```python
from build123d import *

# Parameters (mm, degrees)
F0_R           = 30
F1_DEPTH       = 6
F2_R           = 27
F3_DEPTH       = 0.55
F4_R           = 0.75
F5_DEPTH       = 30.001
F5_DEPTH_BACK  = 30.001
F6_R           = 20
F7_DEPTH       = 5.4510001
F8_R           = 0.75
F9_DEPTH       = 30.0010001
F9_DEPTH_BACK  = 30.0010001
F11_DEPTH      = 3.95
F11_DEPTH_BACK = 0.5510001
F13_DEPTH      = 4.5
F14_R          = 2.05
F15_DEPTH      = 1.5010001


with BuildPart() as f1:
    # F0 (on Top) → F1 (new body)
    with BuildSketch(Plane.XY):
        Circle(F0_R)
    extrude(amount=F1_DEPTH)

    # F2 (on face) → F3 (cut)
    with BuildSketch(Plane.XY.offset(6)):
        Circle(F2_R)
    extrude(amount=-F3_DEPTH, mode=Mode.SUBTRACT)

    # F4 (on Front) → F5 (cut, two sides)
    with BuildSketch(Plane.XZ) as f5_sk:
        with Locations((0, 2.2661738681)):
            Circle(F4_R)
    extrude(amount=-F5_DEPTH, mode=Mode.SUBTRACT)
    extrude(f5_sk.sketch, amount=F5_DEPTH_BACK, mode=Mode.SUBTRACT)

    # F6 (on face) → F7 (cut, through all)
    with BuildSketch(Plane.XY.offset(5.45)):
        Circle(F6_R)
    extrude(amount=-F7_DEPTH, mode=Mode.SUBTRACT)

    # F8 (on Right) → F9 (cut, two sides)
    with BuildSketch(Plane.YZ) as f9_sk:
        with Locations((0, 4)):
            Circle(F8_R)
    extrude(amount=-F9_DEPTH, mode=Mode.SUBTRACT)
    extrude(f9_sk.sketch, amount=F9_DEPTH_BACK, mode=Mode.SUBTRACT)

    # F10 (on face) → F11 (cut, two sides)
    with BuildSketch(Plane.XY.offset(5.45)) as f11_sk:
        with BuildLine():
            ThreePointArc((-24.9057688902, 10.4260575477), (-28.0026498746, 7.54), (-26.7736042577, 3.4891424523))
            ThreePointArc((-26.7736042577, 3.4891424523), (-26.0714326419, 7.02), (-24.9057688902, 10.4260575477))
        make_face()
        with BuildLine():
            ThreePointArc((24.9057688902, -10.4260575477), (26.0714326419, -7.02), (26.7736042577, -3.4891424523))
            ThreePointArc((26.7736042577, -3.4891424523), (20.2777809437, -5.46), (24.9057688902, -10.4260575477))
        make_face()
    extrude(amount=-F11_DEPTH, mode=Mode.SUBTRACT)
    extrude(f11_sk.sketch, amount=F11_DEPTH_BACK, mode=Mode.SUBTRACT)

    # F12 (on face) → F13 (cut)
    with BuildSketch(Plane.XY.offset(6)):
        with BuildLine():
            ThreePointArc((-26.7736042577, 3.4891424523), (-22.4869694193, 2.8576411905), (-20.1402154091, 6.5))
            ThreePointArc((-20.1402154091, 6.5), (-21.5968135459, 9.587249093), (-24.9057688902, 10.4260575477))
            ThreePointArc((-24.9057688902, 10.4260575477), (-28.0026498746, 7.54), (-26.7736042577, 3.4891424523))
        make_face()
        with BuildLine():
            ThreePointArc((26.7736042577, -3.4891424523), (26.0714326419, -7.02), (24.9057688902, -10.4260575477))
            ThreePointArc((24.9057688902, -10.4260575477), (27.2274645021, -9.0434018632), (28.1402154091, -6.5))
            ThreePointArc((28.1402154091, -6.5), (27.7825742186, -4.8467540102), (26.7736042577, -3.4891424523))
        make_face()
    extrude(amount=-F13_DEPTH, mode=Mode.SUBTRACT)

    # F14 (on face) → F15 (cut, through all)
    with BuildSketch(Plane.XY.offset(1.5)):
        with Locations((-24.1402154091, 6.5)):
            Circle(F14_R)
        with Locations((24.1402154091, -6.5)):
            Circle(F14_R)
    extrude(amount=-F15_DEPTH, mode=Mode.SUBTRACT)


solid = f1.part
```
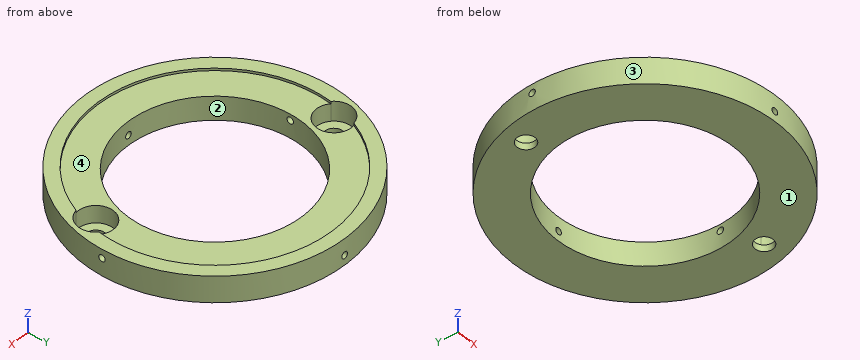
Source: CAD feature listing. Evaluate the final solid. Frame: model axes, mm. Face numbers are marked on the shaded views. Give positions to 0.01 mm unless a question says otherwise; leave off trailing zeros. Write each loop counter-clockwise with the first axis right and the second up, starting at its lowest first coordinate (ties: lowest second). Pieces come first, ordered by that corner, then holes. Notation, with made-up numbers: (62, -22) - (117, -22) arc R25 cw to (117, 12) - close; hole circle Ø2 at (31, -29.5). An arc over 180 degrees is marked (long way). One line per item, written item: value. Start each with the question number.
Q1. First-contact query: pin 1 Ø1.4 at (y, z) = (0, 4) entering from +X; pin 2 Ø3 at (x, z) = (23.5, 2) entering from +Y; pin 3 Ø12 at (x, y) = (19.5, 0.5) entering from +Z; pin 4 Ø2.5 at (x, y) = (22.5, -6) entering from +Z. Flat tips, straight axial feed; report the tip coordinate or a pass-through.
Q2. Section query A-A, the plane x = -4. Return the cut outline in (y, z), then the cut area to 3 significant figures.
Q3. Section query D-D, the plane y = 12. Return the cut outline in (x, z).
Q4. Section query B-B, the plane y = 0. Return the cut outline in (x, z), then the cut area to 3 significant figures.
Q5. Draft query along Y for the marked faces 1, 2, 3 and 4. Return one class per face: +Y half, -Y half, draft (parallel to the pull), parting line (faces both ways), or undercut.
Q6. Material intervals for probe 1 along Z at (x, y) = (26, 0); probe 2 along X at (y, z) = (-6.5, 3.3); probe 3 along X at (y, z) = (-9.5, 2.5), sorted ascending. Write a range as from..to.
Answer:
1. pin 1: passes through
1. pin 2: stops at y = 20.4
1. pin 3: stops at z = 5.45
1. pin 4: stops at z = 1.5
2. outline: (-29.73, 0) - (-19.6, 0) - (-19.6, 5.45) - (-26.7, 5.45) - (-26.7, 6) - (-29.73, 6) - close; (19.6, 0) - (29.73, 0) - (29.73, 6) - (26.7, 6) - (26.7, 5.45) - (19.6, 5.45) - close
2. area: 114 mm2
3. outline: (-27.5, 0) - (-16, 0) - (-16, 5.45) - (-24.19, 5.45) - (-24.19, 6) - (-27.5, 6) - close; (16, 0) - (27.5, 0) - (27.5, 6) - (24.19, 6) - (24.19, 5.45) - (16, 5.45) - close
4. outline: (-30, 0) - (-20, 0) - (-20, 3.25) - (-30, 3.25) - close; (-30, 4.75) - (-20, 4.75) - (-20, 5.45) - (-27, 5.45) - (-27, 6) - (-30, 6) - close; (20, 0) - (30, 0) - (30, 3.25) - (20, 3.25) - close; (20, 4.75) - (30, 4.75) - (30, 6) - (27, 6) - (27, 5.45) - (20, 5.45) - close
4. area: 82.3 mm2
5. face 1: draft
5. face 2: undercut
5. face 3: parting line
5. face 4: undercut
6. probe 1: z = 0..3.25, 4.75..5.45
6. probe 2: x = -29.29..-18.91, 18.91..20.14, 28.14..29.29
6. probe 3: x = -28.46..-17.6, 17.6..21.49, 26.79..28.46
